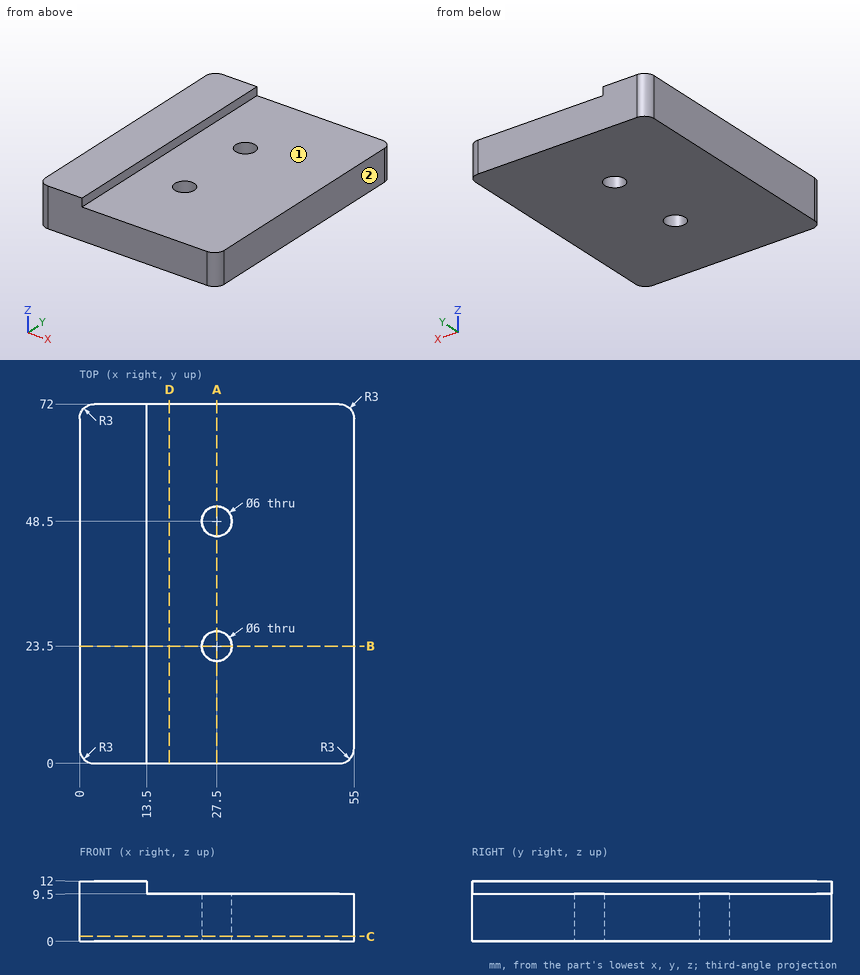
Part print with two shaded views. Sizes in mm from the minimum x, y, z corner. A direction names the side the tool comes from. Round coordinates to 2 decimals unless told otherwise and drop trailing zeros. Write each loop counter-clockwise with the first axis right and the second up, starting at its lowest first coordinate (ties: lowest second). Pieces come first, ordered by that corner, then holes. Notation, with made-up numbers: M 68,5.5 L 116,5.5 A18 ccw 116,14.5 Z; hole C 50,12.25 d5. An arc over 180 degrees is marked long. Put each result on its own line as item: value. Start each with the question number.
1) Drill centre lines: probe 1 along Y at (x, z) = (27.5, 6.25); probe 2 along X at (y, z) = (23.5, 7.5); probe 3 along Y at (x, z) = (29, 9). Where is each one in solid material? Low to high. Write a range as [from, to].
2) Saw through at D-D, the plane x = 18. Write the cut outline in (y, z), and give its area (3 significant figures).
3) Saw through at B-B, the plane y = 23.5. Write the cut outline in (x, z), and give its area (3 significant figures).
4) Saw through at C-C, the plane z = 1. Write the cut outline in (x, y), and give its area (3 significant figures).
5) Pin check, flat tips, straight feed: pin 1 Ø4 at (x, y) = (20.5, 57) entering from -Z; pin 2 Ø3.5 at (x, y) = (27.5, 48.5) entering from -Z; pin 3 Ø0.8 at (y, z) = (47, 10) entering from +X; pin 4 Ø6 at (x, y) = (41.5, 54.5) entering from +Z. Stop position of each tip, or through.
6) Saw through at A-A, the plane x = 27.5. Write the cut outline in (y, z), and give its area (3 significant figures).
7) 3-axis set-ups, long thin cutter, end or side, ignore diameter. For the marked faces 1 and 2: which of +Z, -Z, +X, -X, +Y, -Y reach the whole face in a straight line?
Resolved:
1. probe 1: [0, 20.5], [26.5, 45.5], [51.5, 72]
1. probe 2: [0, 24.5], [30.5, 55]
1. probe 3: [0, 20.9], [26.1, 45.9], [51.1, 72]
2. outline: M 0,0 L 72,0 L 72,9.5 L 0,9.5 Z
2. area: 684 mm²
3. outline: M 0,0 L 24.5,0 L 24.5,9.5 L 13.5,9.5 L 13.5,12 L 0,12 Z; M 30.5,0 L 55,0 L 55,9.5 L 30.5,9.5 Z
3. area: 499 mm²
4. outline: M 0,3 A3 ccw 3,0 L 52,0 A3 ccw 55,3 L 55,69 A3 ccw 52,72 L 3,72 A3 ccw 0,69 Z; hole C 27.5,23.5 d6; hole C 27.5,48.5 d6
4. area: 3,900 mm²
5. pin 1: z = 0
5. pin 2: through
5. pin 3: x = 13.5
5. pin 4: z = 9.5
6. outline: M 0,0 L 20.5,0 L 20.5,9.5 L 0,9.5 Z; M 26.5,0 L 45.5,0 L 45.5,9.5 L 26.5,9.5 Z; M 51.5,0 L 72,0 L 72,9.5 L 51.5,9.5 Z
6. area: 570 mm²
7. face 1: +Z, +X, +Y, -Y
7. face 2: +Z, -Z, +X, +Y, -Y
